Geometry: see drawing. Coordinates: mm, zero at the bounding-box minimum. A direction names the side the tool comes from. Coordinates: 2 decimals unless noted, no trailing zeros. Loops run counter-clockwise (first coordinate to the right, second up) from the corner with the lowest first, then second, coordinate; pieces in that order, holes last. Notation, with made-up numbers: (47, -12.5) -> (80, -12.5) arc R37 ccw to (80, 25.5) -> close; hole circle Ø3 at (12, 27). An arc over 180 degrees is marked (long way). One line per item, written item: value. Start each with the question number.
Item 1: Section query A-A on z = 8. Return loops of the section in (x, y).
Item 2: Section query C-C on x = 27. Return loops of the section in (y, z), then the cut area to 3 significant figures.
Item 3: Contact query for flat-ended pins moving along their axis: pin 1 Ø1 at (x, z) = (37.5, 47.5) entering from -Y; pin 2 Ø12.5 at (x, z) = (39.5, 6) entering from +Y; pin 3 Ø2 at (x, z) = (34.5, 16.5) entering from +Y; pin 4 Ø5 at (x, z) = (39.5, 30.92) entering from +Y. Output: stop coordinate, or through.
Item 4: Ray query, probe 1 along X at (y, z) = (5.7, 49); probe 2 along Y at (x, z) = (46, 13); probe 3 along Y at (x, z) = (9.5, 22.5). Return the intervals inside material, ascending. Write a range as from..to.
Item 5: Section query B-B on x = 14.5. Return loops of the section in (y, z), then the cut area to 3 significant figures.
Item 6: Section query D-D on y = 0.75. Return loops of the section in (x, z), then the cut area to 3 significant figures.
Item 7: Set-up query: the marked faces 1, 2 and 3. Return all of +Z, -Z, +X, -X, +Y, -Y with unobstructed straight access to the full face (end or side cutting, diameter ignored); none if empty.
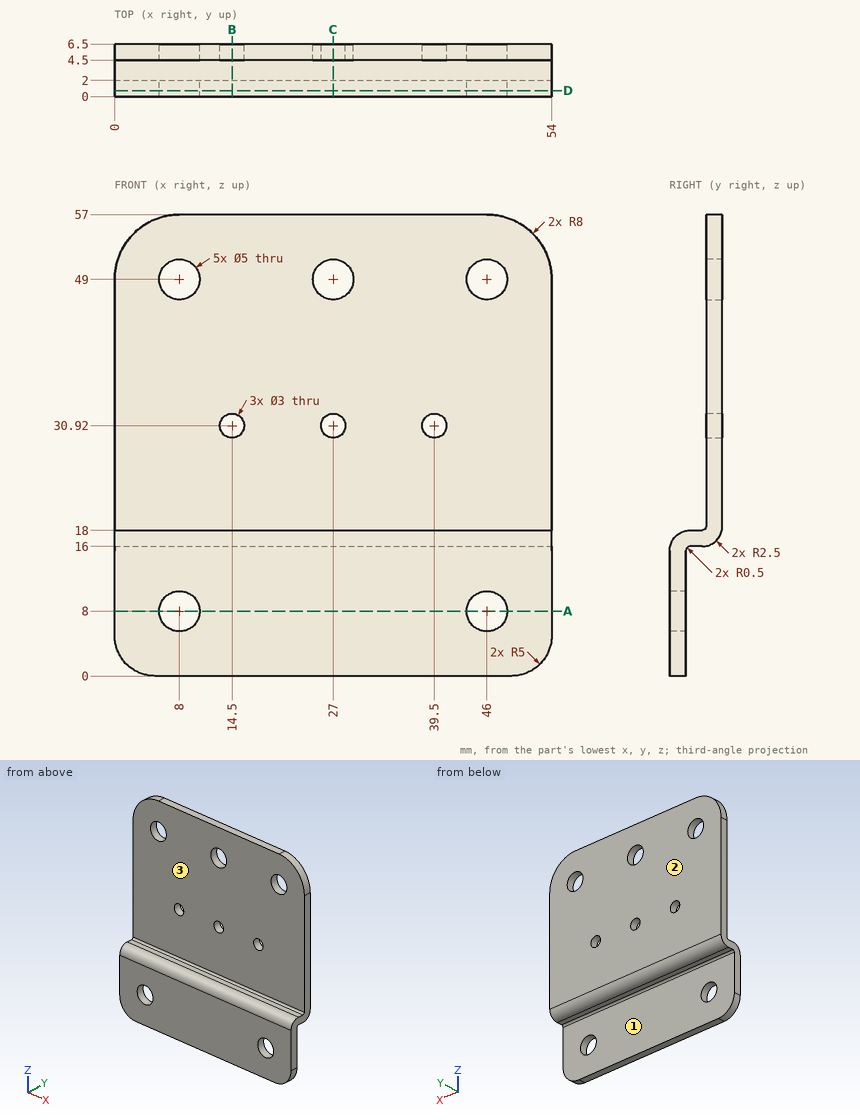
Reply:
1. outline: (0, 0) -> (5.5, 0) -> (5.5, 2) -> (0, 2) -> close; (10.5, 0) -> (43.5, 0) -> (43.5, 2) -> (10.5, 2) -> close; (48.5, 0) -> (54, 0) -> (54, 2) -> (48.5, 2) -> close
2. outline: (0, 0) -> (2, 0) -> (2, 15.5) arc R0.5 cw to (2.5, 16) -> (4, 16) arc R2.5 ccw to (6.5, 18.5) -> (6.5, 29.42) -> (4.5, 29.42) -> (4.5, 18.5) arc R0.5 cw to (4, 18) -> (2.5, 18) arc R2.5 ccw to (0, 15.5) -> close; (4.5, 32.42) -> (6.5, 32.42) -> (6.5, 46.5) -> (4.5, 46.5) -> close; (4.5, 51.5) -> (6.5, 51.5) -> (6.5, 57) -> (4.5, 57) -> close
2. area: 104 mm²
3. pin 1: stops at y = 4.5
3. pin 2: stops at y = 2
3. pin 3: stops at y = 6.29
3. pin 4: stops at y = 6.5
4. probe 1: x = 0..5.5, 10.5..24.5, 29.5..43.5, 48.5..54
4. probe 2: y = 0..2
4. probe 3: y = 4.5..6.5
5. outline: (0, 0) -> (2, 0) -> (2, 15.5) arc R0.5 cw to (2.5, 16) -> (4, 16) arc R2.5 ccw to (6.5, 18.5) -> (6.5, 29.42) -> (4.5, 29.42) -> (4.5, 18.5) arc R0.5 cw to (4, 18) -> (2.5, 18) arc R2.5 ccw to (0, 15.5) -> close; (4.5, 32.42) -> (6.5, 32.42) -> (6.5, 57) -> (4.5, 57) -> close
5. area: 114 mm²
6. outline: (0, 5) arc R5 ccw to (5, 0) -> (49, 0) arc R5 ccw to (54, 5) -> (54, 17.29) -> (0, 17.29) -> close; hole circle Ø5 at (8, 8); hole circle Ø5 at (46, 8)
6. area: 883 mm²
7. face 1: -Z, +X, -X, +Y
7. face 2: +Z, -Z, +X, -X, +Y
7. face 3: +Z, +X, -X, -Y
